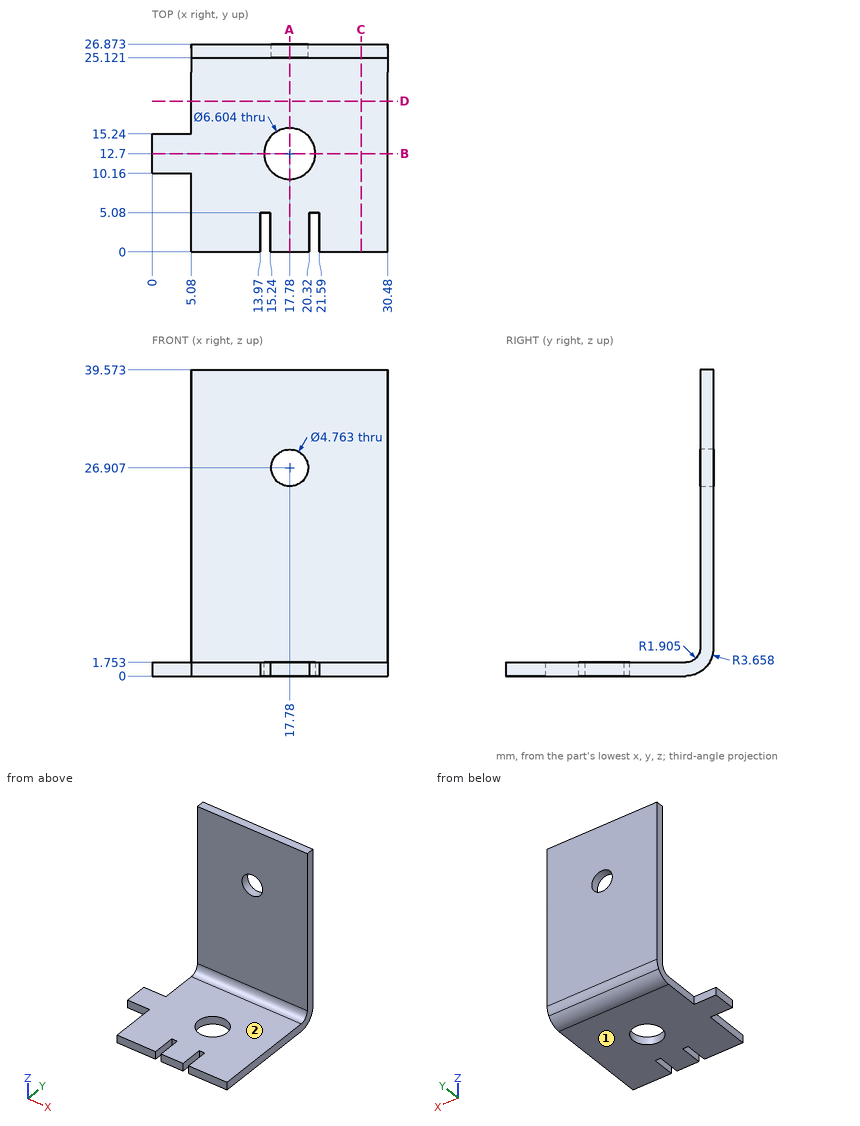
Check sheet for the drawn part. Datum: minimum x, y, z corner. Units: mm. A direction names the side the tool comes from. Round coordinates to 2 decimals unless told otherwise and drop trailing zeros. Loops run counter-clockwise (first coordinate to the right, second up) from the corner with the lowest first, then second, coordinate; pieces in that order, holes last.
Item 1: Cross-section at C-C on x = 27. Record the boundary of the cut face in (y, z) (1 decimal).
Item 2: Thickness scan on line 1 (Y direction, x = 28.5, z = 34); line 2 (Z direction, x = 26, y = 14); line 3 (Y direction, x = 17.78, z = 0.4) (1 decimal). Record the ranges inside material, lowest first.
Item 3: Gauge pin test, flat ends, axial feed: pin 1 (1.5 mm diameter, centred on x = 19, y = 19.5, fed in from +Z); pin 2 (1.9 mm diameter, centred on x = 4, z = 1, fed in from +Y); pin 3 (13 mm diameter, centred on y = 22, z = 10.5, fed in from -X). Record the tip position at first contact, or that the pin passes through.
Item 4: Access from +Z, -Z, +X, -X, +Y, -Y to the whole of each face (thin tool, end or side, straight path). Record for the marked faces 1 and 2.
Item 5: Cross-section at B-B on y = 12.7. Record the boundary of the cut face in (x, z).
Item 6: Cross-section at A-A on x = 17.78. Record the boundary of the cut face in (y, z) (1 decimal).
Item 7: Cross-section at D-D on y = 19.5. Record the boundary of the cut face in (x, z).
Answer sheet:
1. outline: (0, 0) - (23.2, 0) arc R3.7 ccw to (26.9, 3.7) - (26.9, 39.6) - (25.1, 39.6) - (25.1, 3.7) arc R1.9 cw to (23.2, 1.8) - (0, 1.8) - close
2. line 1: y = 25.12 to 26.87
2. line 2: z = 0 to 1.75
2. line 3: y = 0 to 9.4, 16 to 24.9
3. pin 1: stops at z = 1.75
3. pin 2: stops at y = 15.24
3. pin 3: stops at x = 5.08
4. face 1: -Z, +X, -X, +Y, -Y
4. face 2: +Z, +X, -X, -Y
5. outline: (0, 0) - (14.48, 0) - (14.48, 1.75) - (0, 1.75) - close; (21.08, 0) - (30.48, 0) - (30.48, 1.75) - (21.08, 1.75) - close
6. outline: (0, 0) - (9.4, 0) - (9.4, 1.8) - (0, 1.8) - close; (16, 0) - (23.2, 0) arc R3.7 ccw to (26.9, 3.7) - (26.9, 24.5) - (25.1, 24.5) - (25.1, 3.7) arc R1.9 cw to (23.2, 1.8) - (16, 1.8) - close; (25.1, 29.3) - (26.9, 29.3) - (26.9, 39.6) - (25.1, 39.6) - close
7. outline: (5.08, 0) - (30.48, 0) - (30.48, 1.75) - (5.08, 1.75) - close
